Source: CAD feature listing. Evaluate the final solid. Frame: model axes, mm. A direction names the side the tool comes from. Coordinates: 2 decimals unless noted, no trailing zeros. Write each loop counter-clockwise with the first axis right and the second up, starting at its lowest first coordinate (ties: lowest second). Pieces come first, ordered by that corner, then holes. Notation, with made-up numbers: (44.5, 72) -> (78.5, 72) arc R19 cw to (78.5, 85) -> close; hole circle Ø5 at (-10, 89.25). An arc over 180 degrees is marked (long way). One line per item, written item: value. Start each with the question number.
1. Section query A-A, the plane y = 14. Output: boundary loops of the cut face in (x, z), and give its area (3 significant figures).
2. Mould query, pull axis Z, two halves, no side actions, for faces 3 (the flat face through (13, -13, 0)), 4 (the flat face through (0, 25, 42)), 5 (the flat face through (0, 0, -15)). Classes: released by +Z, released by -Z, zero draft, split by the parting line, or undercut.
3. First-contact query: P1, Ø8, axis at x = 9, y = -18, coming from the -Z side. Flat tip, straight axial feed; report the tip coordinate or a pass-through.
4. Section query C-C, the plane x = -14. Output: boundary loops of the cut face in (y, z).
5. Section query D-D, the plane y = -19.5. Output: boundary loops of the cut face in (x, z).
6. Access query for faces 1 (the flat face through (0, 0, 100)), 2 (the flat face through (-5.92, 5.34, -7.4)). Directions: +Z, -Z, +X, -X, +Y, -Y. A direction counts if a zero-diameter tool reaches every point of the face in a straight line with its end or side. Return the directions, or none.
7. Line query: line 1 (Z direction, x = 18, y = 1); line 2 (Y direction, x = 22, z = -5.5); line 3 (Y direction, x = -6, z = -9.5). Output: solid intervals per line, ascending.
8. Section query B-B, the plane x = -4. Output: boundary loops of the cut face in (y, z).
from build123d import *

# Parameters (mm, degrees)
F0_W     = 50
F0_H     = 50
F1_DEPTH = 100
F4_DEPTH = 50
F5_W     = 150
F5_H     = 150
F5_W_2   = 50
F5_H_2   = 50
F6_DEPTH = 15


with BuildPart() as f1:
    # F0 (on Top) → F1 (new body)
    with BuildSketch(Plane.XY):
        Rectangle(F0_W, F0_H)
    extrude(amount=F1_DEPTH)

    # F3 (on 3pt) → F4 (join, symmetric)
    with BuildSketch(Plane(origin=(0, 0, 0), x_dir=(0.7071067812, -0.7071067812, 0), z_dir=(-0.7071067812, -0.7071067812, 0))):
        Polygon((-29.3745769458, 0), (-35.3553390593, 0), (-35.3553390593, -15), (-25.3553390593, -15), align=None)
        Polygon((35.3553390593, -15), (35.3553390593, 0), (29.3745769458, 0), (25.3553390593, -15), align=None)
        Polygon((5.9807621135, 0), (-5.9807621135, 0), (-10, -15), (10, -15), align=None)
    extrude(amount=F4_DEPTH, both=True)

    # F5 (on face) → F6 (cut, through all)
    with BuildSketch(Plane(origin=(0, 0, 0), x_dir=(1, 0, 0), z_dir=(0, 0, -1))):
        Rectangle(F5_W, F5_H)
        Rectangle(F5_W_2, F5_H_2, mode=Mode.SUBTRACT)
    extrude(amount=F6_DEPTH, mode=Mode.SUBTRACT)


solid = f1.part
Computed values:
1. outline: (-25, -15) -> (-21.86, -15) -> (-25, -6.71) -> close; (-25, 0) -> (5.54, 0) -> (-0.14, -15) -> (25, -15) -> (25, -6.71) -> (22.46, 0) -> (25, 0) -> (25, 100) -> (-25, 100) -> close
1. area: 5,340 mm²
2. face 3: undercut
2. face 4: zero draft
2. face 5: released by -Z
3. P1: stops at z = 0
4. outline: (-25, -15) -> (0.14, -15) -> (-5.54, 0) -> (25, 0) -> (25, 100) -> (-25, 100) -> (-25, 0) -> (-22.46, 0) -> (-25, -6.71) -> close; (21.86, -15) -> (25, -15) -> (25, -6.71) -> close
5. outline: (-25, -15) -> (-5.36, -15) -> (-11.04, 0) -> (22.04, 0) -> (16.36, -15) -> (25, -15) -> (25, 100) -> (-25, 100) -> close
6. face 1: +Z, +X, -X, +Y, -Y
6. face 2: none
7. line 1: z = 0 to 100
7. line 2: y = -25 to -17.46, 11.46 to 25
7. line 3: y = -18.06 to 6.06
8. outline: (-25, 0) -> (-12.46, 0) -> (-18.14, -15) -> (10.14, -15) -> (4.46, 0) -> (25, 0) -> (25, 100) -> (-25, 100) -> close
